Could you check a few things on this model? Use its own coordinates, in mm. A direction names the side the tool comes from. Round coordinates to 2 decimals unless told otherwise and drop trailing zeros. Loops run counter-clockwise (first coordinate to the right, second up) from the corner with the lowest first, then second, coordinate; pieces in that order, holes last. Notation, with made-up numbers: M -25,16 L 17,16 A24 cw 17,34 Z; hole C 23,73.5 d9. An arc over 180 degrees is marked long. Answer in a Markdown table with one row per item.
```python
from build123d import *

# Parameters (mm, degrees)
SKETCH1_W                = 28.956
SKETCH1_H                = 26.972
BOSS_EXTRUDE1_DEPTH      = 6.477
BOSS_EXTRUDE1_DEPTH_BACK = 6.477
FILLET1_R                = 1
FILLET2_R                = 1
BOSS_EXTRUDE2_DEPTH      = 2.3
BOSS_EXTRUDE3_DEPTH      = 0.7
FILLET3_R                = 0.3
SKETCH5_R                = 6
BOSS_EXTRUDE4_DEPTH      = 0.7
FILLET4_R                = 0.3
SKETCH6_R                = 4
BOSS_EXTRUDE5_DEPTH      = 5.3
CHAMFER1_SIZE            = 0.5
SKETCH7_R                = 8.5
SKETCH7_R_2              = 4
BOSS_EXTRUDE6_DEPTH      = 1.5
SKETCH8_R                = 0.65
CUT_EXTRUDE1_DEPTH       = 1.5
SKETCH9_R                = 0.65
CUT_EXTRUDE2_DEPTH       = 1.5
CIRPATTERN1_COUNT        = 2
CIRPATTERN1_ANGLE        = 20
CIRPATTERN2_COUNT        = 2
CIRPATTERN2_ANGLE        = 20
CUT_EXTRUDE3_DEPTH       = 0.5
BOSS_EXTRUDE7_DEPTH      = 5.477
BOSS_EXTRUDE7_DEPTH_BACK = 5.477
SKETCH16_W               = 8.954
SKETCH16_H               = 4.011652596
CUT_EXTRUDE4_DEPTH       = 5.055762
SKETCH17_W               = 8.954
SKETCH17_H               = 3.380527785
CUT_EXTRUDE5_DEPTH       = 5.055762
SKETCH18_R               = 2.2
CUT_EXTRUDE6_DEPTH       = 21.941804104


with BuildPart() as part:
    # Sketch1 → Boss-Extrude1 (new body, two sides)
    with BuildSketch(Plane.XY) as boss_extrude1_sk:
        with Locations((0, 0.702144992)):
            Rectangle(SKETCH1_W, SKETCH1_H)
    extrude(amount=BOSS_EXTRUDE1_DEPTH)
    extrude(boss_extrude1_sk.sketch, amount=-BOSS_EXTRUDE1_DEPTH_BACK)

    # Fillet1
    fillet1_edges = [part.edges().sort_by_distance(p)[0] for p in [
        (14.478, 0.702144992, -6.477),
        (-14.478, 0.702144992, 6.477),
        (14.478, 0.702144992, 6.477),
        (-14.478, 0.702144992, -6.477),
    ]]
    fillet(fillet1_edges, radius=FILLET1_R)

    # Fillet2
    fillet2_edges = [part.edges().sort_by_distance(p)[0] for p in [
        (14.478, -12.783855008, 0),
        (0, -12.783855008, -6.477),
        (0, -12.783855008, 6.477),
        (-14.478, -12.783855008, 0),
        (-14.185106781, -12.783855008, 6.184106781),
        (-14.185106781, -12.783855008, -6.184106781),
        (14.185106781, -12.783855008, 6.184106781),
        (14.185106781, -12.783855008, -6.184106781),
    ]]
    fillet(fillet2_edges, radius=FILLET2_R)

    # Sketch3 → Boss-Extrude2 (add)
    with BuildSketch(Plane(origin=(0, 14.188144992, 0), x_dir=(1, 0, 0), z_dir=(0, 1, 0))):
        with BuildLine():
            Line((-10.109849088, 6.477), (8.710547639, 6.477))
            ThreePointArc((8.710547639, 6.477), (9.41765442, 6.184106781), (9.710547639, 5.477))
            Line((9.710547639, 5.477), (9.710547639, 2.882503788))
            ThreePointArc((9.710547639, 2.882503788), (12.593051427, 0), (9.710547639, -2.882503788))
            Line((9.710547639, -2.882503788), (9.710547639, -5.477))
            ThreePointArc((9.710547639, -5.477), (9.41765442, -6.184106781), (8.710547639, -6.477))
            Line((8.710547639, -6.477), (-10.109849088, -6.477))
            ThreePointArc((-10.109849088, -6.477), (-14.478, 0), (-10.109849088, 6.477))
        make_face()
    extrude(amount=BOSS_EXTRUDE2_DEPTH)

    # Sketch4 → Boss-Extrude3 (add)
    with BuildSketch(Plane(origin=(0, 16.488144992, 0), x_dir=(1, 0, 0), z_dir=(0, 1, 0))):
        with BuildLine():
            Line((9.010547639, 2.06720168), (9.010547639, 5.477))
            ThreePointArc((9.010547639, 5.477), (8.922679673, 5.689132034), (8.710547639, 5.777))
            Line((8.710547639, 5.777), (0.524279087, 5.777))
            ThreePointArc((0.524279087, 5.777), (0.312147052, 5.689132034), (0.224279087, 5.477))
            Line((0.224279087, 5.477), (0.224279087, -5.477))
            ThreePointArc((0.224279087, -5.477), (0.312147052, -5.689132034), (0.524279087, -5.777))
            Line((0.524279087, -5.777), (8.710547639, -5.777))
            ThreePointArc((8.710547639, -5.777), (8.922679673, -5.689132034), (9.010547639, -5.477))
            Line((9.010547639, -5.477), (9.010547639, -2.06720168))
            ThreePointArc((9.010547639, -2.06720168), (11.893051427, 0), (9.010547639, 2.06720168))
        make_face()
    extrude(amount=BOSS_EXTRUDE3_DEPTH)

    # Fillet3
    fillet3_edges = [part.edges().sort_by_distance(p)[0] for p in [
        (11.893051427, 17.188144992, 0),
        (9.010547639, 17.188144992, -3.77210084),
        (8.922679673, 17.188144992, -5.689132034),
        (4.617413363, 17.188144992, -5.777),
        (0.312147052, 17.188144992, -5.689132034),
        (0.224279087, 17.188144992, 0),
        (0.312147052, 17.188144992, 5.689132034),
        (4.617413363, 17.188144992, 5.777),
        (8.922679673, 17.188144992, 5.689132034),
        (9.010547639, 17.188144992, 3.77210084),
    ]]
    fillet(fillet3_edges, radius=FILLET3_R)

    # Sketch5 → Boss-Extrude4 (add)
    with BuildSketch(Plane(origin=(0, 16.488144992, 0), x_dir=(1, 0, 0), z_dir=(0, 1, 0))):
        with Locations((-7.491946563, 0)):
            Circle(SKETCH5_R)
    extrude(amount=BOSS_EXTRUDE4_DEPTH)

    # Fillet4
    fillet4_edges = [part.edges().sort_by_distance(p)[0] for p in [
        (-13.491946563, 17.188144992, 0),
    ]]
    fillet(fillet4_edges, radius=FILLET4_R)

    # Sketch6 → Boss-Extrude5 (add)
    with BuildSketch(Plane(origin=(0, 17.188144992, 0), x_dir=(1, 0, 0), z_dir=(0, 1, 0))):
        with Locations((-7.491946563, 0)):
            Circle(SKETCH6_R)
    extrude(amount=BOSS_EXTRUDE5_DEPTH)

    # Chamfer1
    chamfer1_edges = [part.edges().sort_by_distance(p)[0] for p in [
        (-11.491946563, 22.488144992, 0),
    ]]
    chamfer(chamfer1_edges, length=CHAMFER1_SIZE)

    # Sketch7 → Boss-Extrude6 (add)
    with BuildSketch(Plane(origin=(0, 22.488144992, 0), x_dir=(1, 0, 0), z_dir=(0, 1, 0))):
        with Locations((-7.491946563, 0)):
            Circle(SKETCH7_R)
        with Locations((-7.491946563, 0)):
            Circle(SKETCH7_R_2, mode=Mode.SUBTRACT)
    extrude(amount=-BOSS_EXTRUDE6_DEPTH)

    # Sketch8 → Cut-Extrude1 (cut)
    with BuildSketch(Plane(origin=(0, 22.488144992, 0), x_dir=(1, 0, 0), z_dir=(0, 1, 0))):
        with Locations((-7.491946563, -6)):
            Circle(SKETCH8_R)
        with Locations((-7.491946563, 6)):
            Circle(SKETCH8_R)
    extrude(amount=-CUT_EXTRUDE1_DEPTH, mode=Mode.SUBTRACT)

    # Sketch9 → Cut-Extrude2 (cut)
    with BuildSketch(Plane(origin=(0, 22.488144992, 0), x_dir=(1, 0, 0), z_dir=(0, 1, 0))):
        with Locations((-13.991946563, 0)):
            Circle(SKETCH9_R)
        with Locations((-0.991946563, 0)):
            Circle(SKETCH9_R)
    cut_extrude2 = extrude(amount=-CUT_EXTRUDE2_DEPTH, mode=Mode.SUBTRACT)

    # CirPattern1: Cut-Extrude2 ×2 about axis
    cirpattern1_axis = Axis((-7.491946563, 0, 0), (0, 1, 0))
    for i in range(1, CIRPATTERN1_COUNT):
        add(cut_extrude2.rotate(cirpattern1_axis, i * CIRPATTERN1_ANGLE / (CIRPATTERN1_COUNT - 1)), mode=Mode.SUBTRACT)

    # CirPattern2: Cut-Extrude2 ×2 about axis
    cirpattern2_axis = Axis((-7.491946563, 0, 0), (0, -1, 0))
    for i in range(1, CIRPATTERN2_COUNT):
        add(cut_extrude2.rotate(cirpattern2_axis, i * CIRPATTERN2_ANGLE / (CIRPATTERN2_COUNT - 1)), mode=Mode.SUBTRACT)

    # Sketch11 → Revolve1 (revolve)
    with BuildSketch(Plane.XY):
        with BuildLine():
            Line((-4.991946563, 22.488144992), (-4.991946563, 22.888144992))
            add(Edge.make_bspline(
                [(-4.991946563, 22.888144992), (-6.158337638, 23.488144992), (-7.491946563, 23.488144992)],
                knots=[0, 0, 0, 1, 1, 1], degree=2))
            Line((-7.491946563, 23.488144992), (-7.491946563, 22.488144992))
            Line((-7.491946563, 22.488144992), (-4.991946563, 22.488144992))
        make_face()
    revolve(axis=Axis((-7.491946563, 22.488144992, 0), (0, 1, 0)))

    # Sketch12 → Cut-Extrude3 (cut)
    with BuildSketch(Plane(origin=(0, 23.488144992, 0), x_dir=(1, 0, 0), z_dir=(0, 1, 0))):
        Polygon((-7.131090135, -1.285309656), (-7.131090135, -0.360856428), (-6.206636907, -0.360856428), (-6.206636907, 0.360856428), (-7.131090135, 0.360856428), (-7.131090135, 1.285309656), (-7.85280299, 1.285309656), (-7.85280299, 0.360856428), (-8.777256218, 0.360856428), (-8.777256218, -0.360856428), (-7.85280299, -0.360856428), (-7.85280299, -1.285309656), align=None)
    extrude(amount=-CUT_EXTRUDE3_DEPTH, mode=Mode.SUBTRACT)

    # Sketch14 → Boss-Extrude7 (add, two sides)
    with BuildSketch(Plane.XY) as boss_extrude7_sk:
        Polygon((-14.478, 6.012144992), (-19.53376211, 6.012144992), (-19.53376211, 8.157949096), (-17.871474894, 8.157949096), (-16.666917549, 9.936604913), (-14.478, 9.936604913), align=None)
        Polygon((19.53376211, 6.012144992), (19.53376211, 8.157949096), (17.871474894, 8.157949096), (16.666917549, 9.936604913), (14.478, 9.936604913), (14.478, 6.012144992), align=None)
    extrude(amount=BOSS_EXTRUDE7_DEPTH)
    extrude(boss_extrude7_sk.sketch, amount=-BOSS_EXTRUDE7_DEPTH_BACK)

    # Sketch16 → Cut-Extrude4 (cut)
    with BuildSketch(Plane.ZY.offset(19.53376211)):
        with Locations((0, 10.163775394)):
            Rectangle(SKETCH16_W, SKETCH16_H)
    extrude(amount=-CUT_EXTRUDE4_DEPTH, mode=Mode.SUBTRACT)

    # Sketch17 → Cut-Extrude5 (cut)
    with BuildSketch(Plane(origin=(19.53376211, 0, 0), x_dir=(0, 0, -1), z_dir=(1, 0, 0))):
        with Locations((0, 9.848212989)):
            Rectangle(SKETCH17_W, SKETCH17_H)
    extrude(amount=-CUT_EXTRUDE5_DEPTH, mode=Mode.SUBTRACT)

    # Sketch18 → Cut-Extrude6 (cut, through all)
    with BuildSketch(Plane(origin=(0, 8.157949096, 0), x_dir=(1, 0, 0), z_dir=(0, 1, 0))):
        with Locations((17.653, 0)):
            Circle(SKETCH18_R)
        with Locations((-17.653, 0)):
            Circle(SKETCH18_R)
    extrude(amount=-CUT_EXTRUDE6_DEPTH, mode=Mode.SUBTRACT)


solid = part.part
```
1) Which directions (+Z, -Z, +X, -X, +Y, -Y) give clear straight access to the entire face, cutting with the end or side of a thin tool? Please do faces 4 (the face through (-15, 8.158, 0)), 5 (the face through (15, 6.012, 0)), 6 (the face through (-6, 17.188, -4)), 7 (the face through (-15, 6.012, 0)), 8 (the face through (12.592, 15.322, -0.063)).
Computed:
| item | result |
|---|---|
| face 4 | -X |
| face 5 | +Z, -Z, +X, -Y |
| face 6 | none |
| face 7 | +Z, -Z, -X, -Y |
| face 8 | +X, +Y |
2) I need wall thicknesses on line 1 (Y direction, x = -12, z = -0.5); line 2 (X direction, y = 3, z = 3.25); line 3 (X direction, y = 6.75, z = 0). Which ranges of each line are inside material? Lowest first, please.
Computed:
| item | result |
|---|---|
| line 1 | y = -12.78 to 17.19, 20.99 to 22.49 |
| line 2 | x = -14.48 to 14.48 |
| line 3 | x = -15.45 to 15.45 |
3) I want a section at D-D, the plane z = 7.75. Please give me the cut outline in (x, y).
Computed:
| item | result |
|---|---|
| outline | M -10.98,20.99 L -4,20.99 L -4,22.49 L -10.98,22.49 Z |
4) Will these pins go through, and if not, where does the flat tip stop? P1, Ø10, axis at x = 0, z = 4, coming from the +Y side; P2, Ø0.5, axis at x = 15.5, y = 9, coming from the +Z side; P3, Ø5, axis at x = -0.5, y = 12.5, coming from the +Z side; P4, Ø1.5, axis at x = -18, z = 0.5, coming from the +Y side.
Computed:
| item | result |
|---|---|
| P1 | stops at y = 22.49 |
| P2 | stops at z = 5.48 |
| P3 | stops at z = 6.48 |
| P4 | passes through |
5) I want a section at C-C, the plane y = 0. Please give me the cut outline in (x, z).
Computed:
| item | result |
|---|---|
| outline | M -14.48,-5.48 A1 ccw -13.48,-6.48 L 13.48,-6.48 A1 ccw 14.48,-5.48 L 14.48,5.48 A1 ccw 13.48,6.48 L -13.48,6.48 A1 ccw -14.48,5.48 Z |
6) I want a section at B-B, the plane x = 3. Please give me the cut outline in (y, z), plus the area to 3 significant figures.
Computed:
| item | result |
|---|---|
| outline | M -12.78,-5.48 A1 ccw -11.78,-6.48 L 16.49,-6.48 L 16.49,-5.78 L 16.89,-5.78 A0.3 ccw 17.19,-5.48 L 17.19,5.48 A0.3 ccw 16.89,5.78 L 16.49,5.78 L 16.49,6.48 L -11.78,6.48 A1 ccw -12.78,5.48 Z |
| area | 387 mm² |
7) I want a section at A-A, the plane y = 7. Please give me the cut outline in (x, z).
Computed:
| item | result |
|---|---|
| outline | M -19.53,-5.48 L -14.48,-5.48 A1 ccw -13.48,-6.48 L 13.48,-6.48 A1 ccw 14.48,-5.48 L 19.53,-5.48 L 19.53,-1.14 A2.2 cw long 19.53,1.14 L 19.53,5.48 L 14.48,5.48 A1 ccw 13.48,6.48 L -13.48,6.48 A1 ccw -14.48,5.48 L -19.53,5.48 L -19.53,1.14 A2.2 cw long -19.53,-1.14 Z |
8) If we mould it in two halves opening along X, with no side actions, what happens to faces 1 (the face through (-10.67, 19.06, 2.43)), 2 (the face through (15.454, 7.1, -0.08)), 3 (the face through (-14.177, -12.499, -0.077))? For each: released by +X, released by -X, zero draft, split by the parting line, or undercut.
Computed:
| item | result |
|---|---|
| face 1 | split by the parting line |
| face 2 | undercut |
| face 3 | released by -X |
